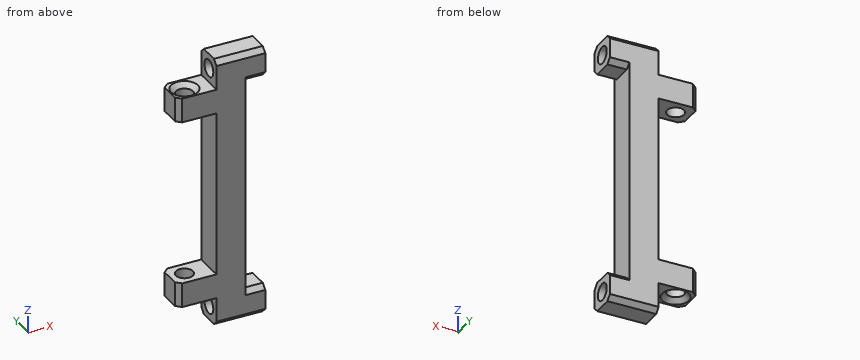
Autodesk Inventor part; units mm, degrees
ref_plane "YZ Plane" through (0, 0, 0) normal (1, 0, 0) x (0, 1, 0)
ref_plane "XZ Plane" through (0, 0, 0) normal (0, 1, 0) x (-1, 0, 0)
ref_plane "XY Plane" through (0, 0, 0) normal (0, 0, 1) x (1, 0, 0)
sketch "Sketch1" plane through (0, 0, 0) normal (0, 1, 0) x (-1, 0, 0)
  line L0 (0, 0) -> (0, -6)
  line L1 (0, -6) -> (4, -6)
  line L2 (4, -6) -> (4, -50)
  line L3 (4, -50) -> (0, -50)
  line L4 (0, -50) -> (0, -56)
  line L5 (0, 0) -> (10, 0)
  line L6 (0, 0) -> (10, 0)
  line L7 (10, 0) -> (10, -6)
  line L8 (10, -6) -> (18, -6)
  line L9 (18, -6) -> (18, -11)
  line L10 (18, -11) -> (10, -11)
  line L11 (10, -11) -> (10, -45)
  line L12 (10, -45) -> (18, -45)
  line L13 (18, -45) -> (18, -50)
  line L14 (18, -50) -> (10, -50)
  line L15 (0, -56) -> (4, -56)
  line L16 (10, -50) -> (10, -56)
  line L17 (10, -56) -> (4, -56)
  point P0 (0, -3)
  point P1 (0, -53)
  dimension "d2" = 50
  dimension "d3" = 6
  dimension "d4" = 4
  dimension "d19" = 6
  dimension "d22" = 8
  dimension "d42" = 6
  dimension "d43" = 6
  dimension "d45" = 5
  dimension "d46" = 34
extrude "Extrusion1" add sketch "Sketch1" along normal blind 6
sketch "Sketch4" plane through (0, 0, -50) normal (1, 0, 0) x (0, 0, -1)
  line L0 (-44, 0) -> (0, 0)
  line L1 (-50, 0) -> (-50, 6)
  line L2 (-44, 0) -> (-50, 6) construction
  circle A0 centre (-47, 3) radius 1.75
  line L3 (0, 0) -> (6, 0)
  line L4 (-44, 6) -> (0, 6)
  line L5 (6, 0) -> (0, 6) construction
  circle A1 centre (3, 3) radius 1.75
  dimension "d24" = 3.5
extrude "Extrusion4" cut sketch "Sketch4" against normal through all
chamfer "Chamfer2" distance 1 angle 45 8 edges at (-2, 6, -6) (-2, 0, -6) (-2, 0, -50) (-2, 6, -50) (-5, 0, -56) (-5, 6, -56) (-5, 6, 0) (-5, 0, 0)
sketch "Sketch5" plane through (-18, 0, -6) normal (0, 0, 1) x (1, 0, 0)
  circle A0 centre (3, 3) radius 3 construction
  line L0 (0, 6) -> (8, 6)
  line L1 (0, 0) -> (0, 6)
  line L2 (0, 0) -> (8, 0)
  circle A1 centre (3, 3) radius 1.75
  point P0 (18, 0)
  dimension "d33" = 3.5
chamfer "Chamfer4" distance 1 angle 45 4 edges at (-18, 0, -47.5) (-18, 6, -47.5) (-18, 0, -8.5) (-18, 6, -8.5)
extrude "Extrusion5" cut sketch "Sketch5" against normal through all
chamfer "Chamfer5" distance 1 angle 45 2 edges at (-16.75, 3, -6) (-16.75, 3, -50)
properties part number "camadapter3"
Build history of the part. All positions in model axes, mm. Give positions to 0.01 mm unless a question says otherwise; leave off trailing zeros. Order: outer loops, then holes, each group sorted by start corner. A loop starts at its lowest first (then second) coordinate and runs counter-clockwise, first axis right, second up. Notation, with made-up numbers: M 34,43.25 L 64,43.25 A18 cw 64,74.25 Z; hole C 75,-10.5 d1. An arc over 180 degrees is marked long. Put each result on its own line as item: value.
Item 1: Flat gauge pins, fed straight in: pin 1 Ø8 at (x, z) = (-2, -6) entering from -Y; pin 2 Ø1.8 at (x, y) = (-14, 3.5) entering from +Z; pin 3 Ø1.8 at (x, y) = (-12.5, 2.5) entering from -Z; pin 4 Ø1 at (y, z) = (2, -22) entering from +X. Where does each tip first touch, or does it go through?
From the geometry:
pin 1: stops at y = 0
pin 2: stops at z = -6.73
pin 3: stops at z = -50
pin 4: stops at x = -4
Item 2: Probe line 1 (Y direction, x = -7.25, z = -3); line 2 (Z direction, x = -8, y = 3.75); line 3 (X direction, y = 5.5, z = -37). List the from-to ranges inside material, lowest first. Write a range as [from, to].
From the geometry:
line 1: y = [0, 1.25], [4.75, 6]
line 2: z = [-56, -54.58], [-51.42, -4.58], [-1.42, 0]
line 3: x = [-10, -4]
Item 3: Slice it at D-D, the plane x = -15. Write the cut outline in (y, z), plus the area to 3 significant figures.
From the geometry:
outline: M 0,-50 L 0.25,-50 L 1.25,-49 L 1.25,-45 L 0,-45 Z; M 0,-11 L 1.25,-11 L 1.25,-7 L 0.25,-6 L 0,-6 Z; M 4.75,-49 L 5.75,-50 L 6,-50 L 6,-45 L 4.75,-45 Z; M 4.75,-11 L 6,-11 L 6,-6 L 5.75,-6 L 4.75,-7 Z
area: 23.0 mm2
Item 4: Slice it at B-B, the plane z = -53. Write the cut outline in (x, y).
From the geometry:
outline: M -10,0 L 0,0 L 0,1.25 L -10,1.25 Z; M -10,4.75 L 0,4.75 L 0,6 L -10,6 Z
Item 5: Slice it at A-A, the plane x = -0.75. Write the cut outline in (y, z).
From the geometry:
outline: M 0,-55 L 1,-56 L 5,-56 L 6,-55 L 6,-51 L 5,-50 L 1,-50 L 0,-51 Z; M 0,-5 L 1,-6 L 5,-6 L 6,-5 L 6,-1 L 5,0 L 1,0 L 0,-1 Z; hole C 3,-53 d3.5; hole C 3,-3 d3.5
Item 6: Slice it at C-C, the plane x = -8. Write the cut outline in (y, z), plus the area to 3 significant figures.
From the geometry:
outline: M 0,-55 L 1,-56 L 5,-56 L 6,-55 L 6,-1 L 5,0 L 1,0 L 0,-1 Z; hole C 3,-53 d3.5; hole C 3,-3 d3.5
area: 315 mm2
